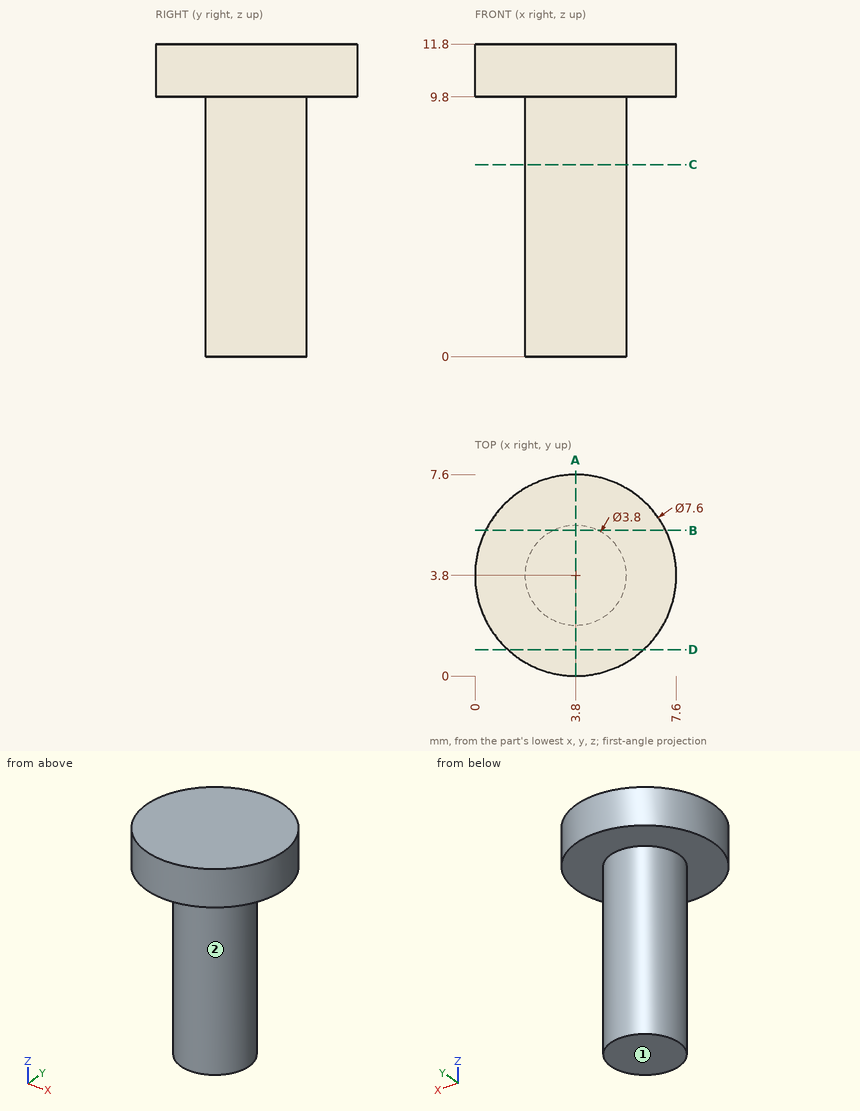
Source: three-view drawing plus pictorial views. Frame: mm from the lowest corner of the part. A direction names the side the tool comes from. Give positions to 0.01 mm unless a question says otherwise; leave off trailing zeros. Loops run counter-clockwise (first coordinate to the right, second up) from the corner with the lowest first, then second, coordinate; pieces in that order, holes last. Notation, with made-up numbers: M 33.25,-11 L 89.25,-11 A21 cw 89.25,21 Z; hole C 60.5,44 d2. An arc over 180 degrees is marked long. Use CSV: the item, a comma, the result in double quotes.
(1) Section B-B, the plane y = 5.5. Return loops of the section in (x, z).
Outcome:
outline,"M 0.4,9.8 L 2.95,9.8 L 2.95,0 L 4.65,0 L 4.65,9.8 L 7.2,9.8 L 7.2,11.8 L 0.4,11.8 Z"
(2) Section C-C, the plane z = 7.25. Return loops of the section in (x, y), plus the area to 3 significant figures.
Outcome:
outline,"C 3.8,3.8 d3.8"
area,"11.3 mm²"
(3) Material intervals for L1, parallel to Z at x = 5.25, y = 2; L2, parallel to Y at x = 3.75, z = 4.75; L3, parallel to Y at x = 3, z = 8, sorted ascending. Write a range as [from, to].
Outcome:
L1,"z = [9.8, 11.8]"
L2,"y = [1.9, 5.7]"
L3,"y = [2.08, 5.52]"
(4) Section D-D, the plane y = 1. Return loops of the section in (x, z), plus the area to 3 significant figures.
Outcome:
outline,"M 1.23,9.8 L 6.37,9.8 L 6.37,11.8 L 1.23,11.8 Z"
area,"10.3 mm²"
(5) Section A-A, the plane x = 3.8. Return loops of the section in (y, z), plus the area to 3 significant figures.
Outcome:
outline,"M 0,9.8 L 1.9,9.8 L 1.9,0 L 5.7,0 L 5.7,9.8 L 7.6,9.8 L 7.6,11.8 L 0,11.8 Z"
area,"52.4 mm²"
(6) Set-up query: the marked faces 1 and 2. Return all of +Z, -Z, +X, -X, +Y, -Y with unobstructed straight access to the full face (end or side cutting, diameter ignored); none if empty.
Outcome:
face 1,"-Z, +X, -X, +Y, -Y"
face 2,"-Z"
(7) Pin query (flat end, axial travel): P1, Ø1, axis at x = 6, z = 1.5, coming from the +Y side; P2, Ø1.5, axis at x = 4, z = 7.5, coming from the -Y side; P3, Ø2.5, axis at x = 4.5, y = 5.5, coming from the -Z side; P4, Ø1.5, axis at x = 2.5, z = 5.5, coming from the -Y side. Return the tip coordinate at first contact, or that it passes through.
Outcome:
P1,"stops at y = 4.65"
P2,"stops at y = 1.9"
P3,"stops at z = 0"
P4,"stops at y = 1.98"
